The model under review builds one solid part; all positions refer to its coordinate system, in mm. A direction names the side the tool comes from. Round coordinates to 2 decimals unless told otherwise and drop trailing zeros. Order: outer loops, then holes, each group sorted by start corner. A loop starts at its lowest first (then second) coordinate and runs counter-clockwise, first axis right, second up. Notation, with made-up numbers: M 8.5,-12 L 65.5,-12 A26 ccw 65.5,5 Z; hole C -2.5,40 d7. An arc over 180 degrees is marked long. Answer as a JSON object with one key per item and string values. Group by question number.
1. Clearance check with flat-ended pins moving along their axes: P1, Ø2, axis at x = 34.5, z = 89, coming from the +Y side; P2, Ø1, axis at y = 19, z = 172.5, coming from the +X side; P3, Ø8, axis at y = 41, z = 81, coming from the -X side; P4, Ø5.5, axis at x = 15, y = -25.98, coming from the -Z side. State where each tip first meets the part, or that it passes through.
2. Machinability: for faces 1 (the face through (-11.503, 25.827, 0.592)), 2 (the face through (6.678, -50.863, 103.67)), which of the approach directions +Z, -Z, +X, -X, +Y, -Y give a long, thin tool a straight path to every point of the face, cutting with its end or side? Answer none if there is none.
3. Add section B-B on z = 178. State the section outline as (x, y) points, and give its area (3 significant figures).
4. To check wall thickness, follow probe 1 along Y at (x, z) = (0.5, 20); probe 2 along Y at (x, z) = (-15, 1); probe 3 along Y at (x, z) = (-8, 83). State the ranges of each line that lie inside material, in increasing order. Write a range as [from, to].
5. Add section C-C on x = -16. Give the number of separate pieces and of enclosed holes in the cut face, and give its area (3 significant figures).
6. Add section A-A on x = 0. State the section outline as (y, z) points, and give its area (3 significant figures).
```python
from build123d import *

# Parameters (mm, degrees)
SKETCH001_R        = 3.5
POCKET_DEPTH       = 698.197748
POLARPATTERN_COUNT = 6


with BuildPart() as part:
    # Sketch → Revolution (revolve)
    with BuildSketch(Plane.XZ):
        with BuildLine():
            Line((0, 0), (-42.5, 0))
            ThreePointArc((-52.5, 10), (-49.571068, 2.928932), (-42.5, 0))
            Line((-52.5, 10), (-52.5, 200))
            Line((-51.3, 200), (-52.5, 200))
            Line((-51.3, 200), (-51.3, 10))
            ThreePointArc((-51.3, 10), (-48.72254, 3.77746), (-42.5, 1.2))
            Line((0, 1.2), (-42.5, 1.2))
            Line((0, 1.2), (0, 0))
        make_face()
    revolve(axis=Axis((0, 0, 0), (0, 0, 1)))

    # Sketch001 → Pocket (cut, through all)
    with BuildSketch(Plane.XY):
        with Locations((-30, 0)):
            Circle(SKETCH001_R)
    pocket = extrude(amount=POCKET_DEPTH, mode=Mode.SUBTRACT)

    # PolarPattern: Pocket ×6 about axis
    polarpattern_axis = Axis((0, 0, 0), (0, 0, 1))
    for i in range(1, POLARPATTERN_COUNT):
        add(pocket.rotate(polarpattern_axis, i * 360 / POLARPATTERN_COUNT), mode=Mode.SUBTRACT)


solid = part.part
```
Recorded:
{
 "1": {"P1": "stops at y = 40.42", "P2": "stops at x = 49.13", "P3": "stops at x = -37.25", "P4": "passes through"},
 "2": {"face 1": "+Z, -Z", "face 2": "+Z"},
 "3": {"outline": "C 0,0 d105; hole C 0,0 d102.6", "area": "391 mm²"},
 "4": {"probe 1": "y = [-52.5, -51.3], [51.3, 52.5]", "probe 2": "y = [-44.39, -29.48], [-22.48, 22.48], [29.48, 44.39]", "probe 3": "y = [-51.89, -50.67], [50.67, 51.89]"},
 "5": {"separate pieces": "3", "enclosed holes": "0", "area": "595 mm²"},
 "6": {"outline": "M -52.5,10 A10 ccw -42.5,0 L 42.5,0 A10 ccw 52.5,10 L 52.5,200 L 51.3,200 L 51.3,10 A8.8 cw 42.5,1.2 L -42.5,1.2 A8.8 cw -51.3,10 L -51.3,200 L -52.5,200 Z", "area": "593 mm²"}
}
